Part model, mm, in its own coordinate system. Coordinates: 2 decimals unless noted, no trailing zeros. Order: outer loops, then holes, each group sorted by start corner. A loop starts at its lowest first (then second) coordinate and runs counter-clockwise, first axis right, second up. Notation, with made-up numbers: M 82.25,19.5 L 139.25,19.5 A38 cw 139.25,58.5 Z; hole C 73.5,8 d6. An arc over 180 degrees is marked long. Answer in a Markdown table with one row per item. Add a question column.
Autodesk Inventor part; units mm, degrees
ref_plane "YZ Plane" through (0, 0, 0) normal (1, 0, 0) x (0, 1, 0)
ref_plane "XZ Plane" through (0, 0, 0) normal (0, 1, 0) x (-1, 0, 0)
ref_plane "XY Plane" through (0, 0, 0) normal (0, 0, 1) x (1, 0, 0)
sketch "Sketch6" plane through (0, 0, 0) normal (0, 1, 0) x (-1, 0, 0)
  line L0 (0, 0) -> (22, 0)
  line L1 (22, 0) -> (22, -22)
  line L2 (22, -22) -> (0, -22)
  line L3 (0, -22) -> (0, 0)
  dimension "d18" = 22
  dimension "d19" = 22
extrude "Extrusion3" add sketch "Sketch6" along normal blind 10
ref_plane "Work Plane1" through (-11, 0, -22) normal (-1, 0, 0) x (0, 0, 1)
sketch "Sketch8" plane through (-11, 0, -22) normal (-1, 0, 0) x (0, 0, 1)
  line L0 (0, 10) -> (22, 10)
  line L1 (11, 10) -> (11, 18)
  circle A0 centre (11, 18) radius 9
  line L2 (11.0985, 9.0005) -> (10.9015, 26.9995)
  point P0 (22, 0)
  dimension "d30" = 8
  dimension "d31" = 18
revolve "Revolution2" add sketch "Sketch8" angle 360 about axis through (-11, 9.0005, -10.9015) along (0, 0.9999401, -0.0109435) picked at (12.4036, 12.6667) picked at (13.3498, 9.8198) contours A0 L0 L2 | L2 L0 A0
properties part number "sphere-test"
(1) Slice it at A-A (x = -17.25). List the corners of the cut face in (y, z).
(2) Slice it at C-C (x = -12). List the corners of the cut face in (y, z).
(3) Drop flat-ended pins along their axis: P1, Ø4, axis at y = 18, z = -12.5, coming from the -X side; P2, Ø12, axis at x = -6, y = 21.5, coming from the -Z side; P3, Ø1.5, axis at y = 12, z = -15.5, coming from the +X side. Give the stop position or say it passes through.
(4) Pull direction Y, two halves, no side cores. Call faces 1 (the flat face through (0, 5, -11)), 2 (the flat face through (-16, 10, -11)), 3 (the flat face through (-11, 0, -11)): pulls with the +Y half, pulls with the -Y half, needs draft (parallel to the pull), parting line crosses it, or undercut.
(5) Wall check: line 1 (Y direction, x = -6.25, z = -12.75); line 2 (Y direction, x = -14, z = -4.5); line 3 (X direction, y = 19.5, z = -6.25). Give the ranges that are in metal, low to high.
(6) Slice it at D-D (z = -14). List the corners of the cut face in (x, y).
(7) Slice it at B-B (z = -16.5). List the corners of the cut face in (x, y).
Computed:
| question | item | result |
|---|---|---|
| 1 | outline | M 0,-22 L 10,-22 L 10,0 L 0,0 Z; C 18,-11 d12.95 |
| 2 | outline | M 0,-22 L 10,-22 L 10,-15 A8.94 ccw long 10,-7 L 10,0 L 0,0 Z |
| 3 | P1 | stops at x = -20 |
| 3 | P2 | stops at z = -20 |
| 3 | P3 | stops at x = -5.05 |
| 4 | face 1 | needs draft |
| 4 | face 2 | undercut |
| 4 | face 3 | pulls with the -Y half |
| 5 | line 1 | y = 0 to 10, 10.56 to 25.44 |
| 5 | line 2 | y = 0 to 10, 12.55 to 23.45 |
| 5 | line 3 | x = -18.5 to -3.5 |
| 6 | outline | M -22,0 L 0,0 L 0,10 L -8.17,10 A8.49 ccw long -13.83,10 L -22,10 Z |
| 7 | outline | M -22,0 L 0,0 L 0,10 L -22,10 Z; C -11,18 d14.25 |
